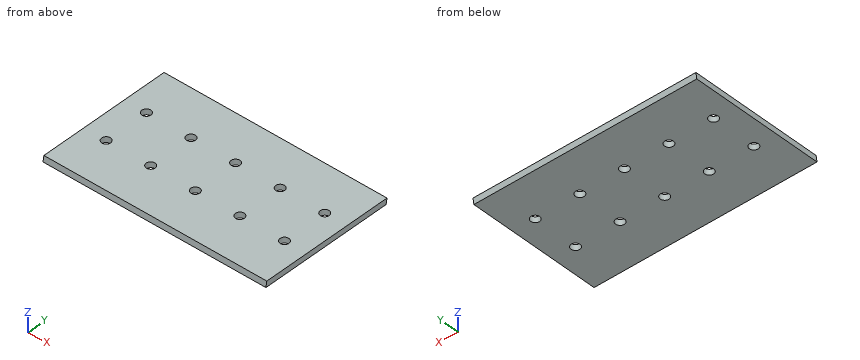
from build123d import *

# Parameters (mm, degrees)
F0_W     = 254
F0_H     = 165.1
F0_R     = 5.08
F1_DEPTH = 6.35
F3_DEPTH = 254.001
F5_DEPTH = 254.001


with BuildPart() as f1:
    # F0 (on Top) → F1 (new body)
    with BuildSketch(Plane.XY):
        with Locations((127, 82.55)):
            Rectangle(F0_W, F0_H)
        with Locations((25.4, 63.881)):
            Circle(F0_R, mode=Mode.SUBTRACT)
        with Locations((76.2, 63.881)):
            Circle(F0_R, mode=Mode.SUBTRACT)
        with Locations((127, 63.881)):
            Circle(F0_R, mode=Mode.SUBTRACT)
        with Locations((177.8, 63.881)):
            Circle(F0_R, mode=Mode.SUBTRACT)
        with Locations((228.6, 63.881)):
            Circle(F0_R, mode=Mode.SUBTRACT)
        with Locations((25.4, 114.681)):
            Circle(F0_R, mode=Mode.SUBTRACT)
        with Locations((76.2, 114.681)):
            Circle(F0_R, mode=Mode.SUBTRACT)
        with Locations((127, 114.681)):
            Circle(F0_R, mode=Mode.SUBTRACT)
        with Locations((177.8, 114.681)):
            Circle(F0_R, mode=Mode.SUBTRACT)
        with Locations((228.6, 114.681)):
            Circle(F0_R, mode=Mode.SUBTRACT)
    extrude(amount=F1_DEPTH)

    # F2 (on face) → F3 (cut, through all)
    with BuildSketch(Plane(origin=(0, 0, 0), x_dir=(0, -1, 0), z_dir=(-1, 0, 0))):
        Polygon((-163.9803236725, 0), (-165.1, 6.35), (-165.1, 0), align=None)
    extrude(amount=-F3_DEPTH, mode=Mode.SUBTRACT)

    # F4 (on face) → F5 (cut, through all)
    with BuildSketch(Plane(origin=(0, 0, 0), x_dir=(0, -1, 0), z_dir=(-1, 0, 0))):
        Polygon((0, 6.35), (-13.462, 6.35), (-12.3423236725, 0), (0, 0), align=None)
        Polygon((0, 0), (-12.3423236725, 0), (19.5333006358, -180.7756486286), (19.5333006358, 6.35), (0, 6.35), align=None)
    extrude(amount=-F5_DEPTH, mode=Mode.SUBTRACT)


solid = f1.part
Here's how the part is built. I have some questions about the finished solid (model axes, mm). Coordinates: 2 decimals unless noted, no trailing zeros. Order: outer loops, then holes, each group sorted by start corner. A loop starts at its lowest first (then second) coordinate and runs counter-clockwise, first axis right, second up. Notation, with made-up numbers: (74.25, 4.25) - (97.25, 4.25) arc R16 cw to (97.25, 34.25) - close; hole circle Ø6 at (38.25, 81.25). An arc over 180 degrees is marked (long way). Use CSV: the item, a comma, the result in double quotes. Start each with the question number.
1. Suppose I cut it at A-A on x = 25.4. List the corners of the cut face in (y, z) for me.
2. Suppose I cut it at B-B on z = 3. Give the number of separate pieces and of enclosed holes in the cut face, then the cut area to 3 significant figures.
3. Please list where these lines run through material, in increasing order: line 1 (Y direction, x = 232.5, z = 1); line 2 (Y direction, x = 25.4, z = 5); line 3 (Y direction, x = 94, z = 1.75). Write a range as from..to.
4. I'm going to push a flat-ended pin straight in: pin 1 (1 mm diameter, centred on x = 160, z = 3, fed in from -Y). Where does the tip first touch, or does it pass through?
Output:
1,outline,"(12.34, 0) - (58.8, 0) - (58.8, 6.35) - (13.46, 6.35) - close; (68.96, 0) - (109.6, 0) - (109.6, 6.35) - (68.96, 6.35) - close; (119.76, 0) - (163.98, 0) - (165.1, 6.35) - (119.76, 6.35) - close"
2,separate pieces,"1"
2,enclosed holes,"10"
2,area,"37,700 mm2"
3,line 1,"y = 12.52..60.63, 67.14..111.43, 117.94..164.16"
3,line 2,"y = 13.22..58.8, 68.96..109.6, 119.76..164.86"
3,line 3,"y = 12.65..164.29"
4,pin 1,"stops at y = 12.78"
